Part model, mm, in its own coordinate system. A direction names the side the tool comes from. Round coordinates to 2 decimals unless told otherwise and drop trailing zeros. Loops run counter-clockwise (first coordinate to the right, second up) from the corner with the lowest first, then second, coordinate; pieces in that order, holes last. Notation, with made-up numbers: (-23, 83) -> (-17, 83) arc R21 ccw to (-17, 99) -> close; hole circle Ø7 at (-29.75, 44). An arc over 180 degrees is marked (long way). Answer as CSV lines item,"result".
from build123d import *

# Parameters (mm, degrees)
SKETCH1_R           = 17.5
SKETCH1_R_2         = 8
SKETCH1_R_3         = 2.75
BOSS_EXTRUDE1_DEPTH = 4
SKETCH1_3_R         = 8
SKETCH1_3_R_2       = 2.75
BOSS_EXTRUDE2_DEPTH = 4
SKETCH1_4_R         = 8
SKETCH1_4_R_2       = 2.75
BOSS_EXTRUDE3_DEPTH = 21
SKETCH2_R           = 5.5
CUT_EXTRUDE1_DEPTH  = 21
SKETCH4_R           = 6
CUT_EXTRUDE2_DEPTH  = 1.1
SKETCH5_R           = 1.5
CUT_EXTRUDE3_DEPTH  = 21.1
CHAMFER1_SIZE       = 0.5


with BuildPart() as part:
    # Sketch1 → Boss-Extrude1 (new body)
    # profile 1 of 3: a face of its own
    with BuildSketch(Plane(origin=(0, 0, 0), x_dir=(1, 0, 0), z_dir=(0, 1, 0))):
        with Locations(Location((0, 0, 0), (0, 0, 270))):
            Circle(SKETCH1_R)
        Circle(SKETCH1_R_2, mode=Mode.SUBTRACT)
    # profile 2 of 3: a face of its own
    with BuildSketch(Plane(origin=(0, 0, 0), x_dir=(1, 0, 0), z_dir=(0, 1, 0))):
        Circle(SKETCH1_R_2)
        Circle(SKETCH1_R_3, mode=Mode.SUBTRACT)
    # profile 3 of 3: a face of its own
    with BuildSketch(Plane(origin=(0, 0, 0), x_dir=(1, 0, 0), z_dir=(0, 1, 0))):
        Circle(SKETCH1_R_3)
    extrude(amount=BOSS_EXTRUDE1_DEPTH)

    # Sketch1_3 → Boss-Extrude2 (add)
    with BuildSketch(Plane(origin=(0, 0, 0), x_dir=(1, 0, 0), z_dir=(0, 1, 0))):
        Circle(SKETCH1_3_R)
        Circle(SKETCH1_3_R_2, mode=Mode.SUBTRACT)
    extrude(amount=BOSS_EXTRUDE2_DEPTH)

    # Sketch1_4 → Boss-Extrude3 (add)
    with BuildSketch(Plane(origin=(0, 0, 0), x_dir=(1, 0, 0), z_dir=(0, 1, 0))):
        with Locations(Location((0, 0, 0), (0, 0, 90))):
            Circle(SKETCH1_4_R)
        with Locations(Location((0, 0, 0), (0, 0, 90))):
            Circle(SKETCH1_4_R_2, mode=Mode.SUBTRACT)
    extrude(amount=BOSS_EXTRUDE3_DEPTH)

    # Sketch2 → Cut-Extrude1 (cut)
    with BuildSketch(Plane(origin=(0, 16, 0), x_dir=(1, 0, 0), z_dir=(0, 1, 0))):
        with Locations(Location((0, 0, 0), (0, 0, 270))):
            Circle(SKETCH2_R)
    extrude(amount=-CUT_EXTRUDE1_DEPTH, mode=Mode.SUBTRACT)

    # Sketch4 → Cut-Extrude2 (cut)
    with BuildSketch(Plane(origin=(0, 13.1, 0), x_dir=(1, 0, 0), z_dir=(0, 1, 0))):
        with Locations(Location((0, 0, 0), (0, 0, 270))):
            Circle(SKETCH4_R)
    extrude(amount=-CUT_EXTRUDE2_DEPTH, mode=Mode.SUBTRACT)

    # Sketch5 → Cut-Extrude3 (cut)
    with BuildSketch(Plane(origin=(0, 4, 0), x_dir=(1, 0, 0), z_dir=(0, 1, 0))):
        with Locations(Location((0, 13, 0), (0, 0, 270))):
            Circle(SKETCH5_R)
        with Locations(Location((13, 0, 0), (0, 0, 270))):
            Circle(SKETCH5_R)
        with Locations(Location((0, -13, 0), (0, 0, 270))):
            Circle(SKETCH5_R)
        with Locations(Location((-13, 0, 0), (0, 0, 270))):
            Circle(SKETCH5_R)
    extrude(amount=-CUT_EXTRUDE3_DEPTH, mode=Mode.SUBTRACT)

    # Chamfer1
    chamfer1_edges = [part.edges().sort_by_distance(p)[0] for p in [
        (0, 21, 8),
        (0, 21, 2.75),
        (0, 0, -17.5),
        (0, 0, -5.5),
        (0, 0, -14.5),
        (13, 0, -1.5),
        (0, 0, 11.5),
        (-13, 0, -1.5),
        (0, 4, -17.5),
    ]]
    chamfer(chamfer1_edges, length=CHAMFER1_SIZE)


solid = part.part
Q1. Saw through at D-D, the plane y = 18.25. Write the cut outline in (x, z).
Geometry results:
outline,"circle Ø16 at (0, 0); hole circle Ø5.5 at (0, 0)"
Q2. Saw through at A-A, the plane z = 0. Give the number of separate pieces and of enclosed holes in the cut face, then the cut area to 3 significant figures.
Geometry results:
separate pieces,"4"
enclosed holes,"0"
area,"182 mm2"
Q3. Two-plate mould, pull along Y, no slides. Class faces 1 (the face through (3, 21, -2)), 2 (the face through (1.802, 12.558, 5.723)), 3 (the face through (-5.37, 14.57, -1.19)): pulls with the +Y half, pulls with the -Y half, needs draft (parallel to the pull), parting line crosses it, or undercut.
Geometry results:
face 1,"pulls with the +Y half"
face 2,"undercut"
face 3,"needs draft"
Q4. Drop flat-ended pins along their axis: P1, Ø3.5, axis at x = 1, z = -2.5, coming from the -Y side; P2, Ø4, axis at x = -13, y = 4.5, coming from the -Z side; P3, Ø4, axis at x = -4, y = 6.5, coming from the -Z side. Give the stop position or say it passes through.
Geometry results:
P1,"y = 16"
P2,"z = -13.39"
P3,"z = -7.75"
Q5. Drill centre lines: line 1 along X through (y, z) = (19.2, 0); line 2 along Y through (x, z) = (-15, 4.5); line 3 along Z through (x, y) = (-0.5, 1.75). Where is each one in solid material? Low to high.
Geometry results:
line 1,"-8 to -2.75, 2.75 to 8"
line 2,"0 to 4"
line 3,"-17.49 to -14.41, -11.59 to -5.48, 5.48 to 11.59, 14.41 to 17.49"
Q6. Which spindle directions (+Z, -Z, +X, -X, +Y, -Y) get a long thin tool onto all of the face, cutting with end or side? Do faces 4 (the face through (2.685, 18.218, 0.596)), 5 (the face through (3, 16, 1)), 6 (the face through (0, 0, -7)), 7 (the face through (7.81, 12.13, 1.73)), 8 (the face through (-5, 12, 3)). Say none if no direction does.
Geometry results:
face 4,"+Y, -Y"
face 5,"-Y"
face 6,"+Z, -Z, +X, -X, -Y"
face 7,"+Y"
face 8,"none"
Q7. Saw through at B-B, the plane y = 8.75. Write the cut outline in (x, z), then the cut area to 3 significant figures.
Geometry results:
outline,"circle Ø16 at (0, 0); hole circle Ø11 at (0, 0)"
area,"106 mm2"
